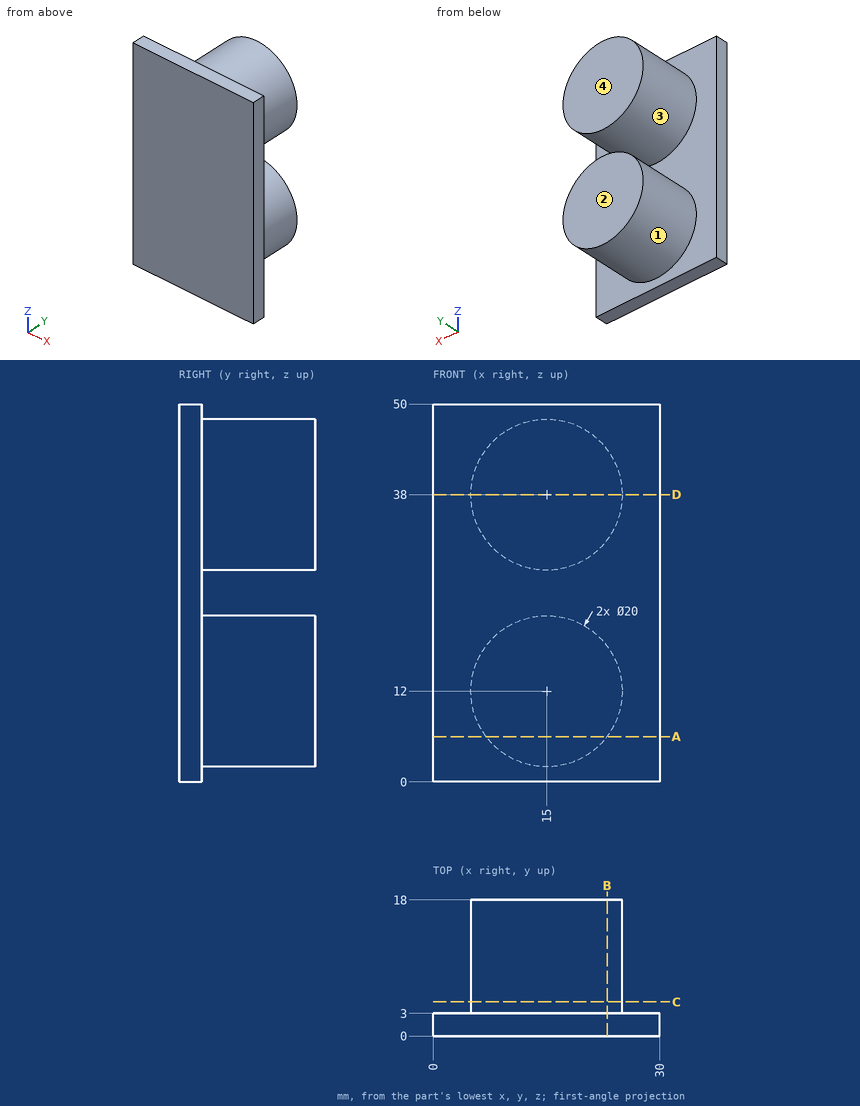
Geometry check sheet. Reference: drawing and pictorial views, mm from the part's lowest x, y, z. A direction names the side the tool comes from. Coordinates: 2 decimals unless noted, no trailing zeros. Write each loop counter-clockwise with the first axis right and the second up, starting at its lowest first coordinate (ties: lowest second). Pieces come first, ordered by that corner, then holes. Notation, with made-up numbers: M 57,-2.75 L 100,-2.75 A9 cw 100,3.25 Z; hole C 82.5,-32 d8. An arc over 180 degrees is marked long. Write item = value, one per line. Start each with the question number.
1. Go/stop test with flat-tipped pins: pin 1 (1.5 mm diameter, centred on x = 18, y = 6, fed in from -Z); pin 2 (3 mm diameter, centred on x = 16, y = 10.5, fed in from -Z); pin 3 (8 mm diameter, centred on y = 10, z = 39.5, fed in from -X). Record where each tip stops, or that it passes through.
2. Sectioned sample at B-B (x = 23). Record the cut outline in (y, z).
3. Thickness scan on probe 1 along Y at (x, z) = (10.75, 23); probe 2 along Z at (x, y) = (23.5, 13.25); probe 3 along Z at (x, y) = (8.25, 13.5). Record the ranges inside material, lowest first.
4. Sectioned sample at C-C (y = 4.5). Record the cut outline in (x, z).
5. Mould release check, pull along Z, two halves, no side actions. Record for the marked faces 3 and 4: pulls with the +Z half, pulls with the -Z half, needs draft (parallel to the pull), parting line crosses it, or undercut.
6. Sectioned sample at D-D (z = 38). Record the cut outline in (x, y), then the cut area to 3 significant figures.
7. Tool access check on the marked faces 1 and 2. Record the directions out of +Z, -Z, +X, -X, +Y, -Y that give a thin tool (end or side, any length) a straight path to the whole face; none if there is none.
8. Sectioned sample at A-A (z = 6). Record the cut outline in (x, y), then the cut area to 3 significant figures.
The answers:
q1.pin_1 = 2.26
q1.pin_2 = 2
q1.pin_3 = 5
q2.outline = M 0,0 L 3,0 L 3,6 L 18,6 L 18,18 L 3,18 L 3,32 L 18,32 L 18,44 L 3,44 L 3,50 L 0,50 Z
q3.probe_1 = 0 to 3
q3.probe_2 = 6.73 to 17.27, 32.73 to 43.27
q3.probe_3 = 4.62 to 19.38, 30.62 to 45.38
q4.outline = C 15,12 d20; C 15,38 d20
q5.face_3 = undercut
q5.face_4 = needs draft
q6.outline = M 0,0 L 30,0 L 30,3 L 25,3 L 25,18 L 5,18 L 5,3 L 0,3 Z
q6.area = 390 mm²
q7.face_1 = +Y
q7.face_2 = +Z, -Z, +X, -X, +Y
q8.outline = M 0,0 L 30,0 L 30,3 L 23,3 L 23,18 L 7,18 L 7,3 L 0,3 Z
q8.area = 330 mm²
